Part model, mm, in its own coordinate system. A direction names the side the tool comes from. Round coordinates to 2 decimals unless told otherwise and drop trailing zeros. Loops run counter-clockwise (first coordinate to the right, second up) from the corner with the lowest first, then second, coordinate; pieces in that order, holes last. Notation, with made-up numbers: (15.25, -31) -> (64.25, -31) arc R15 cw to (64.25, -12) -> close; hole circle Ø11 at (70.5, 84). An arc over 180 degrees is marked (long way). Answer as a JSON object with one key per item and string values. Group by question number.
from build123d import *

# Parameters (mm, degrees)
SKETCH063_W             = 50
SKETCH063_H             = 20
PAD062_DEPTH            = 5
SKETCH064_W             = 50
SKETCH064_H             = 3
PAD063_DEPTH            = 20
SKETCH065_W             = 50
SKETCH065_H             = 10
PAD064_DEPTH            = 3
BODY045_ROLL_ANGLE      = 90
BODY045_PITCH_ANGLE     = 60
BODY045_PLACEMENT_ANGLE = 90


with BuildPart() as part:
    # Sketch063 → Pad062 (new body)
    with BuildSketch(Plane.XY):
        with Locations((184.845276, -123.914059)):
            Rectangle(SKETCH063_W, SKETCH063_H)
    extrude(amount=PAD062_DEPTH)

    # Sketch064 (on Face6 of Pad062) → Pad063 (join)
    with BuildSketch(Plane.XY.offset(5)):
        with Locations((184.83606, -132.417099)):
            Rectangle(SKETCH064_W, SKETCH064_H)
    extrude(amount=PAD063_DEPTH)

    # Sketch065 (on Face7 of Pad063) → Pad064 (join)
    with BuildSketch(Plane(origin=(0, -113.914059, 0), x_dir=(-1, 0, 0), z_dir=(0, 1, 0))):
        with Locations((-184.841869, 9.989668)):
            Rectangle(SKETCH065_W, SKETCH065_H)
    extrude(amount=-PAD064_DEPTH)


with BuildPart() as part_1:
    # Body045 roll: moved
    add(part.part.rotate(Axis((0, 0, 0), (1, 0, 0)), BODY045_ROLL_ANGLE))


with BuildPart() as part_2:
    # Body045 pitch: moved
    add(part_1.part.rotate(Axis((0, 0, 0), (0, 1, 0)), BODY045_PITCH_ANGLE))


with BuildPart() as part_3:
    # Body045 placement: moved
    add(part_2.part.moved(Location((-123, 31.390183, 363.451047))).rotate(Axis((-123, 31.390183, 363.451047), (0, 0, 1)), BODY045_PLACEMENT_ANGLE))


solid = part_3.part
Item 1: Band-saw the part on D-D, the plane x = -101.5. List the corners of the cut face in (y, z), plus the area to 3 significant figures.
Item 2: Drill centre lines: line 1 (X direction, y = 8, z = 161.5); line 2 (Y direction, x = -113, z = 155.5); line 3 (Y direction, x = -114, z = 149). Where is each one in solid material? Low to high.
Item 3: Which spindle directions (+Z, -Z, +X, -X, +Y, -Y) get a long thin tool onto all of the face, cutting with end or side? Do faces 5 (the face through (-108.01, 24, 145)), 6 (the face through (-108.14, 7.66, 136.72)), 7 (the face through (-112.94, 22.736, 144.613)). Say none if no direction does.
Item 4: Two-plate mould, pull along Z, no slides. Class faces 1 (the face through (-118, 16, 142)), 2 (the face through (-113.075, 36.378, 124.026)), 3 (the face through (-113.08, 11.38, 167.33)), 4 (the face through (-98, 9, 137)): pulls with the +Z half, pulls with the -Z half, needs draft (parallel to the pull), parting line crosses it, or undercut.
Item 5: Drop flat-ended pins along their axis: pin 1 Ø1 at (x, z) = (-114, 151.5) entering from -Y; pin 2 Ø10 at (y, z) = (29, 145) entering from +X; pin 3 Ø2 at (x, y) = (-115, 8) entering from -Z. Give the stop position or say it passes through.
Item 6: Band-saw the part on A-A, the plane x = -117.25. List the corners of the cut face in (y, z), plus the area to 3 significant figures.
Entries:
{
 "1": {"outline": "(-4.67, 158.07) -> (20.33, 114.77) -> (22.93, 116.27) -> (-2.07, 159.57) -> close", "area": "150 mm²"},
 "2": {"line 1": "-123 to -118", "line 2": "-3.18 to 0.28, 16.45 to 19.91", "line 3": "0.57 to 4.03, 20.2 to 23.67"},
 "3": {"face 5": "+Z, +X, +Y", "face 6": "-Z, +X, -X, -Y", "face 7": "+X"},
 "4": {"face 1": "undercut", "face 2": "pulls with the -Z half", "face 3": "pulls with the +Z half", "face 4": "needs draft"},
 "5": {"pin 1": "y = -1.16", "pin 2": "x = -108.01", "pin 3": "z = 134.4"},
 "6": {"outline": "(-4.67, 158.07) -> (20.33, 114.77) -> (22.93, 116.27) -> (-2.07, 159.57) -> close; (10.06, 166.57) -> (35.06, 123.27) -> (37.66, 124.77) -> (12.66, 168.07) -> close", "area": "300 mm²"}
}
